Here's how the part is built. I have some questions about the finished solid (model axes, mm). A direction names the side the tool comes from. Coordinates: 2 decimals unless noted, no trailing zeros. Write each loop counter-clockwise with the first axis right and the second up, starting at its lowest first coordinate (ties: lowest second). Pieces come first, ordered by that corner, then holes.
Autodesk Inventor part; units mm, degrees
ref_plane "YZ Plane" through (0, 0, 0) normal (1, 0, 0) x (0, 1, 0)
ref_plane "XZ Plane" through (0, 0, 0) normal (0, 1, 0) x (-1, 0, 0)
ref_plane "XY Plane" through (0, 0, 0) normal (0, 0, 1) x (1, 0, 0)
sketch "スケッチ1" plane through (0, 0, 0) normal (0, 1, 0) x (-1, 0, 0)
  arc A0 (-1.2381, 4.8443) -> (1.2381, 4.8443) centre (0, 0) ccw
  line L0 (1.05, 5.0865) -> (1.05, 8.0865)
  line L1 (1.3, 8.3365) -> (4.8692, 8.3365)
  line L2 (-1.05, 5.0865) -> (-1.05, 8.0865)
  line L3 (-1.3, 8.3365) -> (-4.4822, 8.3365)
  line L4 (-4.7322, 8.0865) -> (-4.7322, 4.8365)
  line L5 (0, 0) -> (0, 8.2759) construction
  arc A1 (1.05, 5.0865) -> (1.2381, 4.8443) centre (1.3, 5.0865) ccw
  arc A2 (-1.2381, 4.8443) -> (-1.05, 5.0865) centre (-1.3, 5.0865) ccw
  arc A3 (-1.7788, -7.0755) -> (1.7788, -7.0755) centre (0, -6.8) ccw
  arc A4 (-4.9679, 4.1916) -> (-5.9354, 2.6497) centre (0, 0) ccw
  arc A5 (2.6497, -5.9354) -> (5.9354, -2.6497) centre (0, 0) ccw
  line L6 (0, -6.8) -> (0, 0) construction
  arc A6 (2.6497, -5.9354) -> (1.7788, -7.0755) centre (3.2611, -7.3051) ccw
  arc A7 (-1.7788, -7.0755) -> (-2.6497, -5.9354) centre (-3.2611, -7.3051) ccw
  circle A8 centre (0, -6.8) radius 0.8
  arc A9 (5.1192, 4.3365) -> (5.3033, 3.7583) centre (6.1192, 4.3365) ccw
  arc A10 (-4.9679, 4.1916) -> (-4.7322, 4.8365) centre (-5.7322, 4.8365) ccw
  line L7 (1.05, 8.0865) -> (1.3, 8.3365)
  line L8 (-1.05, 8.0865) -> (-1.3, 8.3365)
  arc A11 (5.1192, 7.1865) -> (5.1192, 5.9865) centre (5.9192, 6.5865) ccw
  line L9 (5.1192, 8.0865) -> (5.1192, 7.1865)
  line L10 (5.1192, 5.9865) -> (5.1192, 4.3365)
  line L11 (1.05, 6.5865) -> (5.9192, 6.5865) construction
  line L12 (5.1192, 8.0865) -> (4.8692, 8.3365)
  line L13 (-4.7322, 8.0865) -> (-4.4822, 8.3365)
  arc A12 (7.0755, -1.7788) -> (7.0755, 1.7788) centre (6.8, 0) ccw
  arc A13 (6.2684, -1.7197) -> (6.2684, 1.7197) centre (0, 0) ccw construction
  arc A14 (5.9354, 2.6497) -> (5.3033, 3.7583) centre (0, 0) ccw
  circle A15 centre (6.8, 0) radius 0.8
  arc A16 (7.0755, -1.7788) -> (5.9354, -2.6497) centre (7.3051, -3.2611) ccw
  arc A17 (5.9354, 2.6497) -> (7.0755, 1.7788) centre (7.3051, 3.2611) ccw
  line L14 (6.8, 0) -> (0, 0) construction
  arc A18 (-7.0755, 1.7788) -> (-7.0755, -1.7788) centre (-6.8, 0) ccw
  circle A19 centre (-6.8, 0) radius 0.8
  arc A20 (-5.9354, -2.6497) -> (-7.0755, -1.7788) centre (-7.3051, -3.2611) ccw
  arc A21 (-7.0755, 1.7788) -> (-5.9354, 2.6497) centre (-7.3051, 3.2611) ccw
  arc A22 (-5.9354, -2.6497) -> (-2.6497, -5.9354) centre (0, 0) ccw
  arc A23 (-5.9354, 2.6497) -> (-5.9354, -2.6497) centre (0, 0) ccw construction
  point P0 (-1.05, 4.8885)
  point P1 (1.05, 4.8885)
  point P2 (1.05, 8.3365)
  point P3 (5.1192, 8.3365)
  point P4 (5.1192, 4.0055)
  point P5 (-1.05, 8.3365)
  point P6 (-4.7322, 8.3365)
  point P7 (-4.7322, 4.456)
  dimension "d0" = 5
  dimension "d1" = 2.1
  dimension "d2" = 0.25
  dimension "d8" = 6.5
  dimension "d9" = 1.8
  dimension "d11" = 1.5
  dimension "d12" = 1.6
  dimension "d13" = 1
  dimension "d14" = 4
  dimension "d15" = 3.5
  dimension "d16" = 0.25
  dimension "d17" = 0.25
  dimension "d18" = 0.25
  dimension "d19" = 0.25
  dimension "d20" = 3
  dimension "d21" = 1
  dimension "d22" = 0.8
  dimension "d23" = 0.25
  dimension "d24" = 0.25
  dimension "d25" = 0.25
  dimension "d26" = 0.25
  dimension "d27" = 1.5
extrude "押し出し1" add sketch "スケッチ1" along normal blind 4
sketch "スケッチ2" plane through (-5.1192, 0, 7.1865) normal (-1, 0, 0) x (0, 0, 1)
  circle A0 centre (-0.6, 2) radius 1
  line L0 (-0.6, 2) -> (-0.6, 4) construction
  line L1 (-2.1, 4) -> (0.9, 4) construction
  point P0 (-7.1865, 0)
  dimension "d30" = 2
  dimension "d31" = 2
extrude "押し出し2" cut sketch "スケッチ2" against normal blind 10
properties part number "lod_holder" material "アルミニウム 6061"
1) Imagine slicing it at C-C on y = 0.5. Count the separate pieces of the cut face and the enclosed holes in it, then the cut area to 3 significant figures.
Values follow:
separate pieces: 1
enclosed holes: 3
area: 86.1 mm2
2) On a 3-axis mill with a long thin cutter (end or side, diameter ignored), from which of +Z, -Z, +X, -X, +Y, -Y can I reach the whole of each face in a straight line? I mean faces 1 (the face through (-6.386, 1.972, -2.075)), 2 (the face through (-5.119, 2, 5)), 3 (the face through (1.05, 3, 6)). Say none if no direction works.
Values follow:
face 1: -Z, -X, +Y, -Y
face 2: +Z, -X, +Y, -Y
face 3: +Z, +Y, -Y
3) I need wall thicknesses on probe 1 along X at (y, z) = (2.15, 5.25); probe 2 along X at (y, z) = (1.2, -0.5); probe 3 along Z at (x, y) = (0, 2.15). Which ranges of each line are inside material? Lowest first, please.
Values follow:
probe 1: x = -5.12 to -1.05, 1.05 to 4.73
probe 2: x = -8.53 to -7.42, -6.18 to -4.97, 4.97 to 6.18, 7.42 to 8.53
probe 3: z = -8.6 to -7.6, -6 to -5
4) Will these pins go through, and if not, where does the flat tip stop? pin 1 (0.9 mm diameter, centred on y = 2.5, z = 7, fed in from -X); pin 2 (1 mm diameter, centred on x = 6, y = 2, fed in from -Z).
Values follow:
pin 1: stops at x = -5.12
pin 2: stops at z = -3.46
5) We'd pull the mould along Z, two halves only. Please class faces 4 (the face through (-2.063, 1.972, -6.403)), 5 (the face through (0.104, 1.972, -7.593)), 6 (the face through (8.6, 2, 0)), 7 (the face through (-6.403, 1.972, 2.063)): pulls with the +Z half, pulls with the -Z half, needs draft (parallel to the pull), parting line crosses it, or undercut.
Values follow:
face 4: pulls with the -Z half
face 5: undercut
face 6: parting line crosses it
face 7: pulls with the +Z half
6) Imagine slicing it at B-B on x = 0. Please give me the cut outline in (y, z).
Values follow:
outline: (0, -8.6) - (4, -8.6) - (4, -7.6) - (0, -7.6) - close; (0, -6) - (4, -6) - (4, -5) - (0, -5) - close
7) Imagine slicing it at A-A on z = 0. Please give me the cut outline in (x, y), then the cut area to 3 significant figures.
Values follow:
outline: (-8.6, 0) - (-7.6, 0) - (-7.6, 4) - (-8.6, 4) - close; (-6, 0) - (-5, 0) - (-5, 4) - (-6, 4) - close; (5, 0) - (6, 0) - (6, 4) - (5, 4) - close; (7.6, 0) - (8.6, 0) - (8.6, 4) - (7.6, 4) - close
area: 16.0 mm2
